Source: CAD feature listing. Evaluate the final solid. Frame: model axes, mm. Round coordinates to 2 decimals unless told otherwise and drop trailing zeros. Order: outer loops, then holes, each group sorted by start corner. A loop starts at its lowest first (then second) coordinate and runs counter-clockwise, first axis right, second up. Notation, with made-up numbers: M 73.5,-21 L 102.5,-21 A28 cw 102.5,13 Z; hole C -5,47 d5. An arc over 180 degrees is marked long. Answer as CSV lines item,"result". Start each with the question number.
Item 1: First-contact query: P1, Ø1, axis at y = 1, z = 127.5, coming from the -X side; P2, Ø3, axis at x = 1, z = 192, coming from the -Y side; P3, Ø1.5, axis at y = 2.5, z = 64.5, coming from the -X side; P4, Ø2, axis at x = 2, z = 178, coming from the -Y side. Flat tips, straight axial feed; report the tip coordinate or a pass-through.
Item 2: Line query: line 1 (Y direction, x = -0.25, z = 370.5); line 2 (X direction, y = -0.5, z = 166); line 3 (Y direction, x = -3.5, z = 134.5). Output: solid intervals per line, ascending. Write a range as [from, to].
Item 3: Section query A-A on z = 378.5. Return the cut outline in (x, y).
Autodesk Inventor part; units mm, degrees
ref_plane "YZ Plane" through (0, 0, 0) normal (1, 0, 0) x (0, 1, 0)
ref_plane "XZ Plane" through (0, 0, 0) normal (0, 1, 0) x (-1, 0, 0)
ref_plane "XY Plane" through (0, 0, 0) normal (0, 0, 1) x (1, 0, 0)
sketch "Skizze1" plane through (0, 0, 0) normal (0, 0, 1) x (1, 0, 0)
  line L0 (-5.6, 0) -> (5.6, 0)
  line L1 (0, -5.6) -> (0, 5.6)
  circle A0 centre (0, 0) radius 4
  dimension "d0" = 8
extrude "Extrusion1" add sketch "Skizze1" along normal blind 420
thread "Gewinde1"
chamfer "Fase1" distance 0.5 angle 45 1 edges at (-4, 0, 420)
chamfer "Fase2" distance 0.5 angle 45 1 edges at (-4, 0, 0)
properties part number "Gewindestange_M8x420mm"
Results:
1,P1,"x = -3.97"
1,P2,"y = -4"
1,P3,"x = -3.6"
1,P4,"y = -3.87"
2,line 1,"[-3.99, 3.99]"
2,line 2,"[-3.97, 3.97]"
2,line 3,"[-1.94, 1.94]"
3,outline,"C 0,0 d8"
